from build123d import *

# Parameters (mm, degrees)
BOSS_EXTRUDE1_DEPTH     = 7.8994
CUT_EXTRUDE1_DEPTH      = 132.627694139
CUT_EXTRUDE1_DEPTH_BACK = 132.627694139
CUT_EXTRUDE2_DEPTH      = 112.485808354
CUT_EXTRUDE2_DEPTH_BACK = 112.485808354
M6X1_0_TAPPED_HOLE1_D   = 5


with BuildPart() as part:
    # Sketch1 → Boss-Extrude1 (new body)
    with BuildSketch(Plane.XY):
        Polygon((-101.6, 83.312), (-101.6, 38.1), (-69.85, 38.1), (-31.75, 38.1), (0, 38.1), (0, 83.312), align=None)
    extrude(amount=BOSS_EXTRUDE1_DEPTH)

    # Sketch2 → Cut-Extrude1 (cut, two sides: drawn at the far end of the back side and taken through both)
    with BuildSketch(Plane.ZY.offset(101.6).offset(-CUT_EXTRUDE1_DEPTH_BACK)):
        Polygon((59.566381815, 133.911082828), (7.8994, 72.376195004), (5.022457184, 68.949783256), (7.8994, 66.534195004), (69.434287825, 14.867213189), (229.583733305, 28.142484569), (219.715827295, 147.186354208), align=None)
    extrude(amount=CUT_EXTRUDE1_DEPTH + CUT_EXTRUDE1_DEPTH_BACK, mode=Mode.SUBTRACT)

    # Sketch3 → Cut-Extrude2 (cut, two sides: drawn at the far end of the back side and taken through both)
    with BuildSketch(Plane(origin=(0, 83.312, 0), x_dir=(1, 0, 0), z_dir=(0, 1, 0)).offset(-CUT_EXTRUDE2_DEPTH_BACK)):
        Polygon((35.981993731, -91.760393731), (-47.879, -7.8994), (-50.8, -4.9784), (-53.721, -7.8994), (-137.581993731, -91.760393731), (-137.581993731, -328.955103109), (35.981993731, -328.955103109), align=None)
    extrude(amount=CUT_EXTRUDE2_DEPTH + CUT_EXTRUDE2_DEPTH_BACK, mode=Mode.SUBTRACT)

    # M6x1.0 Tapped Hole1 (through all)
    with Locations(Plane(origin=(-50.8, 0, 0), x_dir=(-1, 0, 0), z_dir=(0, 0, -1))):
        with Locations((-30.795161674, 53.586240129), (29.387245779, 53.586240129)):
            Hole(M6X1_0_TAPPED_HOLE1_D / 2)


solid = part.part
Build history of the part. All positions in model axes, mm. A direction names the side the tool comes from. Give positions to 0.01 mm unless a question says otherwise; leave off trailing zeros. Order: outer loops, then holes, each group sorted by start corner. A loop starts at its lowest first (then second) coordinate and runs counter-clockwise, first axis right, second up. Notation, with made-up numbers: M -4.75,-11.75 L 47.25,-11.75 A29 cw 47.25,20.25 Z; hole C -12.5,58.5 d2. An arc over 180 degrees is marked long. Put each result on its own line as item: value.
Item 1: Probe line 1 (X direction, y = 52, z = 5.5); line 2 (X direction, y = 66.5, z = 5.5); line 3 (Y direction, x = -16, z = 6.75). List the from-to ranges inside material, lowest first. Write a range as [from, to].
From the geometry:
line 1: x = [-101.6, -82.12], [-78.25, -51.32], [-50.28, -21.94], [-18.07, 0]
line 2: x = [-101.6, -51.32], [-50.28, 0]
line 3: y = [38.1, 67.5], [71.01, 83.31]
Item 2: Slice it at A-A, the plane x = -36. Write the cut outline in (y, z), plus the area to 3 significant figures.
From the geometry:
outline: M 38.1,0 L 83.31,0 L 83.31,7.9 L 72.38,7.9 L 68.95,5.02 L 66.53,7.9 L 38.1,7.9 Z
area: 349 mm2
Item 3: Slice it at B-B, the plane y = 55. Write the cut outline in (x, z).
From the geometry:
outline: M -101.6,0 L -82.25,0 L -82.25,7.9 L -101.6,7.9 Z; M -78.13,0 L -22.07,0 L -22.07,7.9 L -47.88,7.9 L -50.8,4.98 L -53.72,7.9 L -78.13,7.9 Z; M -17.94,0 L 0,0 L 0,7.9 L -17.94,7.9 Z
Item 4: 3-axis set-ups, long thin cutter, end or side, ignore diameter. For faces 5 (the flat face through (-52.24, 60.39, 6.42)), 6 (the flat face through (-24, 78, 7.899)), 7 (the flat face through (-75.87, 67.76, 6.44)): which of +Z, -Z, +X, -X, +Y, -Y reach the whole face in a straight line?
From the geometry:
face 5: +Z, +Y, -Y
face 6: +Z, +X, -X, +Y, -Y
face 7: +Z, +X, -X
Item 5: Slice it at C-C, the plane y = 70.5. Write the cut outline in (x, z), plus the area to 3 significant figures.
From the geometry:
outline: M -101.6,0 L 0,0 L 0,6.32 L -49.45,6.32 L -50.8,4.98 L -52.15,6.32 L -101.6,6.32 Z
area: 641 mm2
Item 6: Two-plate mould, pull along X, no slides. Class faces 1 (the flat face through (-101.6, 61, 4)), 2 (the flat face through (0, 60, 4)), 3 (the flat face through (-49.32, 60.39, 6.46)), 4 (the flat face through (-25.023, 70.687, 6.481)): +X half, -X half, draft (parallel to the pull), parting line (faces both ways), or undercut.
From the geometry:
face 1: -X half
face 2: +X half
face 3: undercut
face 4: draft
